from build123d import *

# Parameters (mm, degrees)
SKETCH1_R           = 11.5
BOSS_EXTRUDE2_DEPTH = 5


with BuildPart() as part:
    # Sketch1 → Boss-Extrude2 (new body)
    with BuildSketch(Plane.XY):
        with BuildLine():
            ThreePointArc((2.384173399, 21.820911092), (0, 23), (-2.384173399, 21.820911092))
            ThreePointArc((-2.384173399, 21.820911092), (-17.761952084, 6.72401264), (-36.761417585, -3.445192388))
            Line((-36.761417585, -3.445192388), (-61.264901468, -12.363731157))
            Line((-61.264901468, -12.363731157), (-61.502328705, -12.434243309))
            ThreePointArc((-61.502328705, -12.434243309), (-64.87860936, -18.628180071), (-58.700669217, -22.033643218))
            Line((-58.700669217, -22.033643218), (-30.863510665, -14.051466451))
            ThreePointArc((-30.863510665, -14.051466451), (-20.452273896, -13.332100428), (-10.654478564, -16.925781711))
            ThreePointArc((-10.654478564, -16.925781711), (0, -20), (10.654478564, -16.925781711))
            ThreePointArc((10.654478564, -16.925781711), (20.452273896, -13.332100428), (30.863510665, -14.051466451))
            Line((30.863510665, -14.051466451), (58.700669217, -22.033643218))
            ThreePointArc((58.700669217, -22.033643218), (64.87860936, -18.628180071), (61.502328705, -12.434243309))
            Line((61.502328705, -12.434243309), (61.264901468, -12.363731157))
            Line((61.264901468, -12.363731157), (36.761417585, -3.445192388))
            ThreePointArc((36.761417585, -3.445192388), (17.761952084, 6.72401264), (2.384173399, 21.820911092))
        make_face()
        Circle(SKETCH1_R, mode=Mode.SUBTRACT)
    extrude(amount=BOSS_EXTRUDE2_DEPTH)


solid = part.part
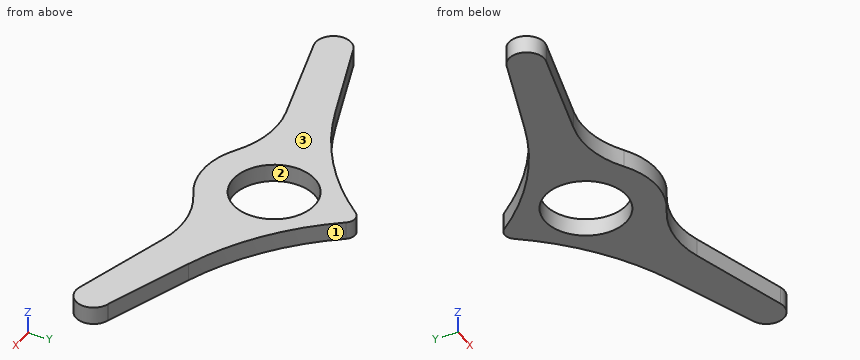
The listing builds one solid part. Answer for the finished solid, in the listing's coordinates (mm). Face numbers are marked on the shaded views. Give positions to 0.01 mm unless a question says otherwise; leave off trailing zeros. Write each loop counter-clockwise with the first axis right and the second up, starting at its lowest first coordinate (ties: lowest second). Pieces come first, ordered by that corner, then holes.
1) Find the intervals of material crossed by L1, parallel to Y at x = 0, z = 3.6; L2, parallel to X at y = 1.5, z = 1.55; L3, parallel to Y at x = -6, z = 3.3, in increasing order.
2) Section D-D (x = -20) is taken. Write down the section's boundary in (y, z), and give its area (3 significant figures).
3) Given P1, Ø1, axis at x = -8.5, z = 1.5, coming from the -Y side; P2, Ø1, axis at y = -1, z = 2.5, coming from the +X side, each flat-ended and moving along its own axis, determine where each tip first touches the part or whether it passes through.
4) Section A-A (x = 0) is taken. Write down the section's boundary in (y, z), and give its area (3 significant figures).
5) Section B-B (y = 2) is taken. Write down the section's boundary in (x, z), and give its area (3 significant figures).
6) For a pull along X with two mould halves and no side action, classify the marked faces 1, 2 and 3 as pulls with the +X half, pulls with the -X half, needs draft (parallel to the pull), parting line crosses it, or undercut.
7) Section C-C (z = 2.3) is taken. Write down the section's boundary in (x, y), and give its area (3 significant figures).
Response:
1. L1: y = -20 to -11.5, 11.5 to 23
1. L2: x = -25.91 to -11.4, 11.4 to 25.91
1. L3: y = -19.08 to -9.81, 9.81 to 17.44
2. outline: (-13.4, 0) - (5.14, 0) - (5.14, 5) - (-13.4, 5) - close
2. area: 92.7 mm2
3. P1: stops at y = -18.33
3. P2: stops at x = 31.94
4. outline: (-20, 0) - (-11.5, 0) - (-11.5, 5) - (-20, 5) - close; (11.5, 0) - (23, 0) - (23, 5) - (11.5, 5) - close
4. area: 100 mm2
5. outline: (-25.02, 0) - (-11.32, 0) - (-11.32, 5) - (-25.02, 5) - close; (11.32, 0) - (25.02, 0) - (25.02, 5) - (11.32, 5) - close
5. area: 137 mm2
6. face 1: pulls with the +X half
6. face 2: undercut
6. face 3: needs draft
7. outline: (-61.5, -12.43) arc R5 ccw to (-58.7, -22.03) - (-30.86, -14.05) arc R25 cw to (-10.65, -16.93) arc R20 ccw to (10.65, -16.93) arc R25 cw to (30.86, -14.05) - (58.7, -22.03) arc R5 ccw to (61.5, -12.43) - (61.26, -12.36) - (36.76, -3.45) arc R75.94 cw to (2.38, 21.82) arc R3 ccw to (-2.38, 21.82) arc R75.94 cw to (-36.76, -3.45) - (-61.26, -12.36) - close; hole circle Ø23 at (0, 0)
7. area: 1,910 mm2
